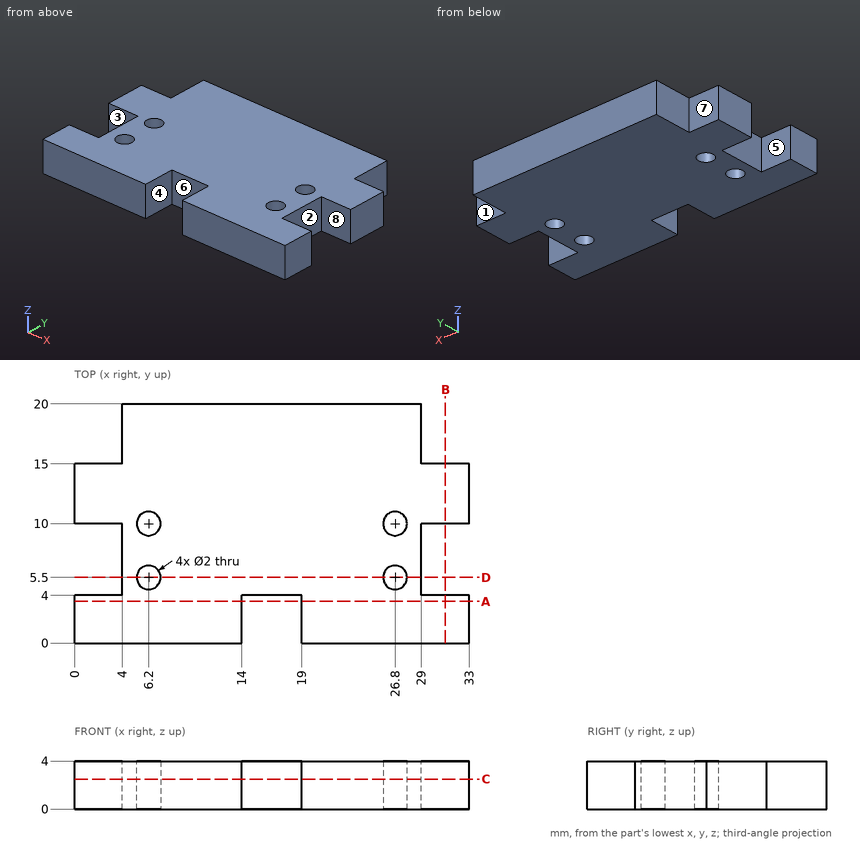
Geometry check sheet. Reference: drawing and pictorial views, mm from the part's lowest x, y, z. A direction names the side the tool comes from. Round coordinates to 2 decimals unless told otherwise and drop trailing zeros. Order: outer loops, then holes, each group sorted by start corner. A loop starts at its lowest first (then second) coordinate and runs counter-clockwise, first axis right, second up. Notation, with made-up numbers: (-11, -37.75) -> (7, -37.75) arc R21 ccw to (7, -31.75) -> close; hole circle Ø1 at (-15, 33). An arc over 180 degrees is marked (long way). One line per item, written item: value. Start each with the question number.
Q1. Thickness scan on line 1 (Y direction, x = 26.8, z = 3.1); line 2 (X direction, y = 1, z = 1); line 3 (X direction, y = 10.5, z = 0.6). Record the ranges inside material, lowest first.
Q2. Gauge pin test, flat ends, axial feed: pin 1 Ø1.2 at (y, z) = (6.5, 2) entering from -X; pin 2 Ø1.2 at (y, z) = (17.5, 1) entering from +X; pin 3 Ø2 at (x, z) = (1, 1) entering from +Y. Record the tip position at first contact, or that the pin passes through.
Q3. Cross-section at B-B (x = 31). Record the boundary of the cut face in (y, z).
Q4. Cross-section at A-A (y = 3.5). Record the boundary of the cut face in (x, z).
Q5. Cross-section at C-C (z = 2.5). Record the boundary of the cut face in (x, y).
Q6. Cross-section at D-D (y = 5.5). Record the boundary of the cut face in (x, z).
Q7. Mould release check, pull along Y, two halves, no side actions. Record for the marked faces 5, 6, 7 and 8: pulls with the +Y half, pulls with the -Y half, needs draft (parallel to the pull), parting line crosses it, or undercut.
Q8. Set-up check for the marked faces 1, 2, 3 and 4: record each of +Z, -Z, +X, -X, +Y, -Y from which the full face is reachable in a straight line by a thin tool's end or side.
Completed:
1. line 1: y = 0 to 4.5, 6.5 to 9, 11 to 20
1. line 2: x = 0 to 14, 19 to 33
1. line 3: x = 0 to 5.33, 7.07 to 25.93, 27.67 to 33
2. pin 1: stops at x = 4
2. pin 2: stops at x = 29
2. pin 3: stops at y = 15
3. outline: (0, 0) -> (4, 0) -> (4, 4) -> (0, 4) -> close; (10, 0) -> (15, 0) -> (15, 4) -> (10, 4) -> close
4. outline: (0, 0) -> (14, 0) -> (14, 4) -> (0, 4) -> close; (19, 0) -> (33, 0) -> (33, 4) -> (19, 4) -> close
5. outline: (0, 0) -> (14, 0) -> (14, 4) -> (19, 4) -> (19, 0) -> (33, 0) -> (33, 4) -> (29, 4) -> (29, 10) -> (33, 10) -> (33, 15) -> (29, 15) -> (29, 20) -> (4, 20) -> (4, 15) -> (0, 15) -> (0, 10) -> (4, 10) -> (4, 4) -> (0, 4) -> close; hole circle Ø2 at (6.2, 5.5); hole circle Ø2 at (6.2, 10); hole circle Ø2 at (26.8, 5.5); hole circle Ø2 at (26.8, 10)
6. outline: (4, 0) -> (5.2, 0) -> (5.2, 4) -> (4, 4) -> close; (7.2, 0) -> (25.8, 0) -> (25.8, 4) -> (7.2, 4) -> close; (27.8, 0) -> (29, 0) -> (29, 4) -> (27.8, 4) -> close
7. face 5: undercut
7. face 6: pulls with the -Y half
7. face 7: pulls with the +Y half
7. face 8: undercut
8. face 1: +Z, -Z, +X, +Y
8. face 2: +Z, -Z, +X
8. face 3: +Z, -Z, -X
8. face 4: +Z, -Z, -Y
